Verification items for the finished model (mm, model axes). Face numbers are marked on the shaded views. A direction names the side the tool comes from. Give positions to 0.01 mm unless a question says otherwise; leave off trailing zeros. Loops run counter-clockwise (first coordinate to the right, second up) from the corner with the lowest first, then second, coordinate; pieces in that order, holes last. Notation, with made-up numbers: M 13,-15.75 L 40,-15.75 A23 ccw 40,-6.75 Z; hole C -17,40.5 d2. An arc over 180 degrees is marked long. Use CSV: the item, a comma, the result in double quotes.
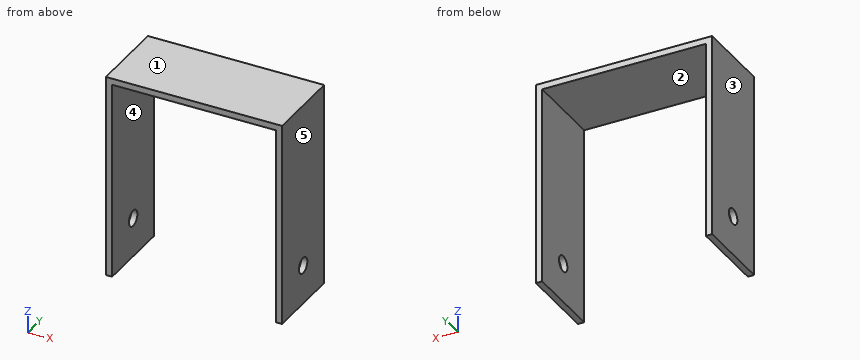
from build123d import *

# Parameters (mm, degrees)
F1_DEPTH      = 12.5
F2_R          = 2.5
F3_DEPTH      = 56.001
F3_DEPTH_BACK = 126


# Not quite as in the source:
# - an extrude ends at something that could not be found from the text; its depth is read off the source's solid


with BuildPart() as f1:
    # F0 (on Front) → F1 (new body, symmetric)
    with BuildSketch(Plane.XZ):
        Polygon((-2, -65), (0, -65), (0, 0), (-56, 0), (-56, -65), (-54, -65), (-54, -2), (-2, -2), align=None)
    extrude(amount=F1_DEPTH, both=True)

    # F2 (on Right) → F3 (cut, two sides)
    with BuildSketch(Plane.YZ) as f3_sk:
        with Locations((0, -52.5)):
            Circle(F2_R)
    extrude(amount=-F3_DEPTH, mode=Mode.SUBTRACT)
    extrude(f3_sk.sketch, amount=F3_DEPTH_BACK, mode=Mode.SUBTRACT)


solid = f1.part
(1) Scan lines: L1, parallel to X at y = -1.5, z = -42; L2, parallel to Z at x = -54.9, y = 0; L3, parallel to Z at x = -49, y = 11. Record each from-to range of solid material in increasing order. Write a range as from..to.
Calculated:
L1,"x = -56..-54, -2..0"
L2,"z = -65..-55, -50..0"
L3,"z = -2..0"
(2) Section check A-A on z = -20.5. Record the cut outline in (x, y), plus the area to 3 significant figures.
Calculated:
outline,"M -56,-12.5 L -54,-12.5 L -54,12.5 L -56,12.5 Z; M -2,-12.5 L 0,-12.5 L 0,12.5 L -2,12.5 Z"
area,"100 mm²"
(3) Section check D-D on x = -30.5. Record the cut outline in (y, z).
Calculated:
outline,"M -12.5,-2 L 12.5,-2 L 12.5,0 L -12.5,0 Z"
(4) Mould release check, pull along X, two halves, no side actions. Record for the marked faces 3, 4 and 5: released by +X, released by -X, zero draft, split by the parting line, or undercut.
Calculated:
face 3,"released by -X"
face 4,"undercut"
face 5,"released by +X"
(5) Section check B-B on y = 0. Record the cut outline in (x, z).
Calculated:
outline,"M -56,-65 L -54,-65 L -54,-55 L -56,-55 Z; M -56,-50 L -54,-50 L -54,-2 L -2,-2 L -2,-50 L 0,-50 L 0,0 L -56,0 Z; M -2,-65 L 0,-65 L 0,-55 L -2,-55 Z"
(6) Depth check by flat-ended pin: pin 1 Ø7.5 at (x, y) = (-35, -0.5) entering from -Z; pin 2 Ø3 at (y, z) = (0, -52.5) entering from -X. Enter the tip coordinate at first touch or a pass-through.
Calculated:
pin 1,"stops at z = -2"
pin 2,"passes through"
(7) Tool access check on the marked faces 1 and 2. Record the directions out of +Z, -Z, +X, -X, +Y, -Y that give a thin tool (end or side, any length) a straight path to the whole face; none if there is none.
Calculated:
face 1,"+Z, +X, -X, +Y, -Y"
face 2,"-Z, +Y, -Y"
(8) Section check C-C on z = -52.5. Record the cut outline in (x, y), plus the area to 3 significant figures.
Calculated:
outline,"M -56,-12.5 L -54,-12.5 L -54,-2.5 L -56,-2.5 Z; M -56,2.5 L -54,2.5 L -54,12.5 L -56,12.5 Z; M -2,-12.5 L 0,-12.5 L 0,-2.5 L -2,-2.5 Z; M -2,2.5 L 0,2.5 L 0,12.5 L -2,12.5 Z"
area,"80.0 mm²"
